Geometry: final body of the model. Coordinates: model frame, mm. A direction names the side the tool comes from. Coordinates: 2 decimals unless noted, no trailing zeros. Loops run counter-clockwise (first coordinate to the right, second up) from the corner with the lowest first, then second, coordinate; pieces in that order, holes last. Notation, with made-up numbers: (-36.5, 71.25) - (-11.5, 71.25) arc R22 cw to (-11.5, 82.25) - close; hole circle Ø5 at (81, -26). An arc over 180 degrees is marked (long way). Return JSON: item names as keys, results as strings.
from build123d import *

# Parameters (mm, degrees)
F0_W      = 25.4
F0_H      = 25.4
F1_DEPTH  = 2.54
F2_W      = 3.4710424952
F2_H      = 3.81
F2_W_2    = 3.81
F3_DEPTH  = 25.4
F4_W      = 3.8600380808
F4_H      = 25.4
F5_DEPTH  = 25.4
F6_W      = 21.5399619192
F6_H      = 4.318
F7_DEPTH  = 3.81
F8_R      = 2.15899
F9_W      = 21.5399619192
F9_H      = 4.318
F10_DEPTH = 3.81
F11_R     = 2.159
F12_R     = 2.15899


# Not quite as in the source:
# - a fillet or chamfer is up to 0.001 mm smaller than in the source, because OpenCascade refuses the exact size


with BuildPart() as f1:
    # F0 (on Top) → F1 (new body)
    with BuildSketch(Plane.XY):
        with Locations((12.7, 12.7)):
            Rectangle(F0_W, F0_H)
    extrude(amount=F1_DEPTH)

    # F2 (on face) → F3 (join)
    with BuildSketch(Plane(origin=(0, 0, 0), x_dir=(1, 0, 0), z_dir=(0, 0, -1))):
        with Locations((1.7355212476, -1.905)):
            Rectangle(F2_W, F2_H)
        with Locations((23.495, -1.905)):
            Rectangle(F2_W_2, F2_H)
        with Locations((1.7355212476, -23.495)):
            Rectangle(F2_W, F2_H)
        with Locations((23.495, -23.495)):
            Rectangle(F2_W_2, F2_H)
    extrude(amount=F3_DEPTH)

    # F4 (on face) → F5 (join)
    with BuildSketch(Plane.XY.offset(2.54)):
        with Locations((23.4699809596, 12.7)):
            Rectangle(F4_W, F4_H)
    extrude(amount=F5_DEPTH)

    # F6 (on face) → F7 (join)
    with BuildSketch(Plane.XY.offset(2.54)):
        with Locations((10.7699809596, 23.241)):
            Rectangle(F6_W, F6_H)
    extrude(amount=F7_DEPTH)

    # F8 (radius 2.159 in the source; OpenCascade refuses exactly that, so slightly less here)
    f8_edges = [f1.edges().sort_by_distance(p)[0] for p in [
        (10.769981, 25.4, 6.35),
        (10.769981, 21.082, 6.35),
    ]]
    fillet(f8_edges, radius=F8_R)

    # F9 (on face) → F10 (join)
    with BuildSketch(Plane.XY.offset(2.54)):
        with Locations((10.7699809596, 2.159)):
            Rectangle(F9_W, F9_H)
    extrude(amount=F10_DEPTH)

    # F11
    f11_edges = [f1.edges().sort_by_distance(p)[0] for p in [
        (10.769981, 0, 6.35),
    ]]
    fillet(f11_edges, radius=F11_R)

    # F12 (radius 2.159 in the source; OpenCascade refuses exactly that, so slightly less here)
    f12_edges = [f1.edges().sort_by_distance(p)[0] for p in [
        (10.769981, 4.318, 6.35),
    ]]
    fillet(f12_edges, radius=F12_R)


solid = f1.part
Item 1: Ray query, probe 1 along Z at (x, y) = (10.75, 11.5); probe 2 along X at (y, z) = (21.25, 23); probe 3 along Z at (x, y) = (22.5, 12). Return the intervals inside material, ascending. Write a range as from..to.
Worked out:
{"probe 1": "0..2.54", "probe 2": "21.54..25.4", "probe 3": "0..27.94"}
Item 2: Mould query, pull axis Y, two halves, no side actions, for faces 1 (the face through (11, 21.082, 3)), 2 (the face through (15, 0, 1)), 3 (the face through (21.59, 24, -13)). Classes: +Y half, -Y half, draft (parallel to the pull), parting line (faces both ways), or undercut.
Worked out:
{"face 1": "undercut", "face 2": "-Y half", "face 3": "draft"}
Item 3: Reachability of faces 4 (the face through (10.921, 0.616, 5.701)), 5 (the face through (3.471, 2, -13)), 6 (the face through (11, 4.318, 3)), 7 (the face through (10.921, 24.784, 5.701)) from +Z, -Z, +X, -X, +Y, -Y: full face, straight path, thin tool, end or side. Return the list, or none.
Worked out:
{"face 4": "+Z, -X, -Y", "face 5": "-Z, +Y, -Y", "face 6": "+Z, -X", "face 7": "+Z, -X, +Y"}
Item 4: Section query A-A, the plane z = -4.5. Return loops of the section in (x, y).
Worked out:
{"outline": "(0, 0) - (3.47, 0) - (3.47, 3.81) - (0, 3.81) - close; (0, 21.59) - (3.47, 21.59) - (3.47, 25.4) - (0, 25.4) - close; (21.59, 0) - (25.4, 0) - (25.4, 3.81) - (21.59, 3.81) - close; (21.59, 21.59) - (25.4, 21.59) - (25.4, 25.4) - (21.59, 25.4) - close"}
Item 5: Section query D-D, the plane z = 9. Return loops of the section in (x, y).
Worked out:
{"outline": "(21.54, 0) - (25.4, 0) - (25.4, 25.4) - (21.54, 25.4) - close"}
Item 6: First-contact query: pin 1 Ø6 at (x, y) = (11, 20.5) entering from +Z; pin 2 Ø2 at (x, z) = (19, -10.5) entering from +Y; pin 3 Ø7.5 at (y, z) = (13, 19) entering from -X; pin 4 Ø6 at (x, y) = (18.5, 3) entering from -Z. Flat tips, straight axial feed; report the tip coordinate or a pass-through.
Worked out:
{"pin 1": "z = 6.35", "pin 2": "through", "pin 3": "x = 21.54", "pin 4": "z = 0"}
Item 7: Section query C-C, the plane y = 12.5. Return loops of the section in (x, z).
Worked out:
{"outline": "(0, 0) - (25.4, 0) - (25.4, 27.94) - (21.54, 27.94) - (21.54, 2.54) - (0, 2.54) - close"}
